The model under review builds one solid part; all positions refer to its coordinate system, in mm. Face numbers are marked on the shaded views. A direction names the side the tool comes from. Coordinates: 2 decimals unless noted, no trailing zeros. Write each loop counter-clockwise with the first axis right and the second up, starting at its lowest first coordinate (ties: lowest second). Pieces come first, ordered by that corner, then holes.
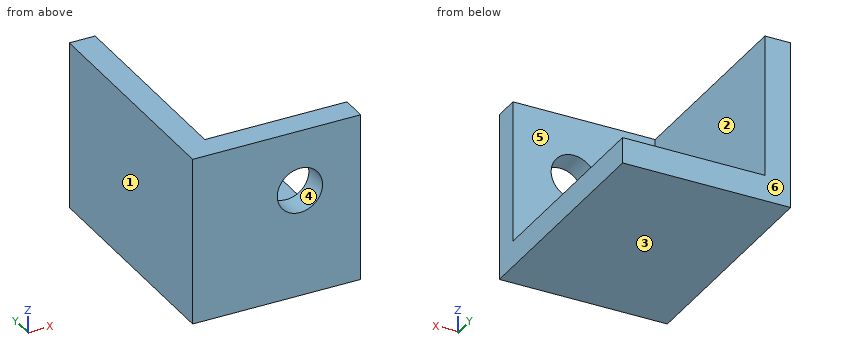
```python
from build123d import *

# Parameters (mm, degrees)
SKETCH1_W           = 13
SKETCH1_H           = 13
BOSS_EXTRUDE1_DEPTH = 2
BOSS_EXTRUDE2_DEPTH = 16
SKETCH3_R           = 1.75
CUT_EXTRUDE1_DEPTH  = 20


with BuildPart() as part:
    # Sketch1 → Boss-Extrude1 (new body)
    with BuildSketch(Plane(origin=(0, 0, 0), x_dir=(1, 0, 0), z_dir=(0, 1, 0))):
        Rectangle(SKETCH1_W, SKETCH1_H)
    extrude(amount=BOSS_EXTRUDE1_DEPTH)

    # Sketch2 → Boss-Extrude2 (add)
    with BuildSketch(Plane(origin=(0, 2, 0), x_dir=(1, 0, 0), z_dir=(0, 1, 0))):
        Polygon((-6.5, 6.5), (-6.5, -6.5), (-4.5, -6.5), (-4.5, 4.5), (6.5, 4.5), (6.5, 6.5), align=None)
    extrude(amount=BOSS_EXTRUDE2_DEPTH)

    # Sketch3 → Cut-Extrude1 (cut)
    with BuildSketch(Plane(origin=(0, 2, 0), x_dir=(1, 0, 0), z_dir=(0, 1, 0))):
        with Locations(Location((1.8, -1.8, 0), (0, 0, 270))):
            Circle(SKETCH3_R)
    extrude(amount=-CUT_EXTRUDE1_DEPTH, mode=Mode.SUBTRACT)


solid = part.part
```
Item 1: Machinability: for the marked faces 5 and 6, which of the approach directions +Z, -Z, +X, -X, +Y, -Y give a long, thin tool a straight path to every point of the face, cutting with its end or side? Answer none if there is none.
Solved:
face 5: +Z, +X, +Y
face 6: +Z, -Z, +X, -X, +Y
Item 2: For pin 1 (3.5 mm diameter, centred on y = 13, z = -0.5, fed in from +X); pin 2 (4 mm diameter, centred on x = -1, z = -1.5, fed in from -Y); pin 3 (4 mm diameter, centred on x = 1.8, z = 1.8, fed in from +Y); pin 4 (3.5 mm diameter, centred on x = 1.5, y = 12, fed in from +Z), all flat-tipped, find the tip position at first contact; note any pin that passes through.
Solved:
pin 1: stops at x = -4.5
pin 2: stops at y = 0
pin 3: stops at y = 2
pin 4: stops at z = -4.5
Item 3: Mouldability with a two-part tool opening along X and no side actions: class the marked faces 1, 2, 3 and 4 as pulls with the +X half, pulls with the -X half, needs draft (parallel to the pull), parting line crosses it, or undercut.
Solved:
face 1: pulls with the -X half
face 2: pulls with the +X half
face 3: needs draft
face 4: undercut
Item 4: Take a section at B-B, the plane z = 0.75. Write out the cut boundary in (x, y), plus the area to 3 significant figures.
Solved:
outline: (-6.5, 0) - (0.4, 0) - (0.4, 2) - (-4.5, 2) - (-4.5, 18) - (-6.5, 18) - close; (3.2, 0) - (6.5, 0) - (6.5, 2) - (3.2, 2) - close
area: 52.4 mm2
Item 5: Take a section at D-D, the plane y = 16.5. Write out the cut boundary in (x, z).
Solved:
outline: (-6.5, -6.5) - (6.5, -6.5) - (6.5, -4.5) - (-4.5, -4.5) - (-4.5, 6.5) - (-6.5, 6.5) - close
Item 6: To check wall thickness, follow line 1 along X through (y, z) = (0.75, 1.8); line 2 along Y through (x, z) = (-2.75, -3.25); line 3 along X through (y, z) = (8.5, -0.75). State the ranges of each line that lie inside material, in increasing order.
Solved:
line 1: x = -6.5 to 0.05, 3.55 to 6.5
line 2: y = 0 to 2
line 3: x = -6.5 to -4.5
Item 7: Take a section at C-C, the plane x = -3. Write out the cut boundary in (y, z), plus the area to 3 significant figures.
Solved:
outline: (0, -6.5) - (18, -6.5) - (18, -4.5) - (2, -4.5) - (2, 6.5) - (0, 6.5) - close
area: 58.0 mm2
Item 8: Take a section at A-A, the plane x = 1.8. Write out the cut boundary in (y, z).
Solved:
outline: (0, -6.5) - (18, -6.5) - (18, -4.5) - (2, -4.5) - (2, 0.05) - (0, 0.05) - close; (0, 3.55) - (2, 3.55) - (2, 6.5) - (0, 6.5) - close
